```python
from build123d import *

# Parameters (mm, degrees)
F0_W        = 30
F0_H        = 10
F1_DEPTH    = 10
F2_R        = 5
F3_T1_DEPTH = 84.348882825
F4_R        = 10
F5_R        = 50
F6_SIZE     = 2
F8_DEPTH    = 10.001
F9_SIZE     = 2


# Not quite as in the source:
# - a fillet or chamfer that OpenCascade refuses, or shapes differently, is made with other operations: its cross-section is extruded or revolved along the edge and cut away or added


with BuildPart() as f1:
    # F0 (on Top) → F1 (new body)
    with BuildSketch(Plane.XY):
        Polygon((5, 50), (-5, 50), (-15, 65), (-15, 75), (-25, 75), (-25, 61.9722436227), (-5, 31.9722436227), (-5, -50), (5, -50), (5, 31.9722436227), (25, 61.9722436227), (25, 75), (15, 75), (15, 65), align=None)
        with Locations((0, 70)):
            Rectangle(F0_W, F0_H)
    extrude(amount=F1_DEPTH)

    # F2
    f2_edges = [f1.edges().sort_by_distance(p)[0] for p in [
        (15, 65, 5),
        (-15, 65, 5),
        (-5, 50, 5),
        (5, 50, 5),
    ]]
    fillet(f2_edges, radius=F2_R)

    # F3: fillet of radius 15 on 2 edges, made by hand

    # F3_s2 → F3_t1 (cut)
    with BuildSketch(Plane.XY.offset(-37.1744414125)):
        with BuildLine():
            ThreePointArc((-25, 61.9722436227), (-20.0149678844, 71.2823679771), (-10.130223435, 75))
            Line((-10.130223435, 75), (-25, 75))
            Line((-25, 75), (-25, 61.9722436227))
        make_face()
        with BuildLine():
            ThreePointArc((25, 61.9722436227), (20.0149678844, 71.2823679771), (10.130223435, 75))
            Line((10.130223435, 75), (25, 75))
            Line((25, 75), (25, 61.9722436227))
        make_face()
    extrude(amount=F3_T1_DEPTH, mode=Mode.SUBTRACT)

    # F4
    f4_edges = [f1.edges().sort_by_distance(p)[0] for p in [
        (-25, 61.972244, 5),
        (25, 61.972244, 5),
    ]]
    fillet(f4_edges, radius=F4_R)

    # F5
    f5_edges = [f1.edges().sort_by_distance(p)[0] for p in [
        (5, 31.972244, 5),
        (-5, 31.972244, 5),
    ]]
    fillet(f5_edges, radius=F5_R)

    # F6
    f6_edges = [f1.edges().sort_by_distance(p)[0] for p in [
        (0, 65, 10),
        (0, 75, 10),
        (0, 50, 0),
        (0, 75, 0),
    ]]
    chamfer(f6_edges, length=F6_SIZE)

    # F7 (on face) → F8 (cut, through all)
    with BuildSketch(Plane.XY.offset(10)):
        Polygon((0, 37.3431457505), (2.8284271247, 40.1715728753), (0, 43), (-2.8284271247, 40.1715728753), align=None)
    extrude(amount=-F8_DEPTH, mode=Mode.SUBTRACT)

    # F9
    f9_edges = [f1.edges().sort_by_distance(p)[0] for p in [
        (1.414214, 41.585786, 10),
        (-1.414214, 41.585786, 10),
        (1.414214, 38.757359, 10),
        (-1.414214, 38.757359, 10),
        (1.414214, 38.757359, 0),
        (1.414214, 41.585786, 0),
        (-1.414214, 41.585786, 0),
        (-1.414214, 38.757359, 0),
    ]]
    chamfer(f9_edges, length=F9_SIZE)


solid = f1.part
```
Geometry: final body of the model. Coordinates: model frame, mm. A direction names the side the tool comes from. Round coordinates to 2 decimals unless told otherwise and drop trailing zeros. Order: outer loops, then holes, each group sorted by start corner. A loop starts at its lowest first (then second) coordinate and runs counter-clockwise, first axis right, second up. Notation, with made-up numbers: (60, 23.5) -> (80, 23.5) arc R13 ccw to (80, 34.5) -> close; hole circle Ø4 at (-25, 13). An arc over 180 degrees is marked (long way). Use one line per item in the form item = value.
(1) Ray query, probe 1 along X at (y, z) = (-9, 4); probe 2 along Y at (x, z) = (-9, 8.5); probe 3 along X at (y, z) = (57, 4). Return the intervals inside material, ascending. Write a range as [from, to].
Results list:
probe_1 = [-5, 5]
probe_2 = [37.67, 55.1], [64.37, 74.5]
probe_3 = [-21.69, -9.67], [9.67, 21.69]
(2) Section B-B on y = -3.5. Return loops of the section in (x, z).
Results list:
outline = (-5, 2) -> (-3, 0) -> (3, 0) -> (5, 2) -> (5, 8) -> (3, 10) -> (-3, 10) -> (-5, 8) -> close
(3) Draft query along X for faces 1 (the face through (23.845, 64.085, 5.042)), 2 (the face through (-6.69, 31.68, 1.46)), 3 (the face through (2.23, 37.86, 0.79)). Return one class per face: pulls with the +X half, pulls with the -X half, needs draft (parallel to the pull), parting line crosses it, or undercut.
Results list:
face_1 = pulls with the +X half
face_2 = pulls with the -X half
face_3 = undercut
(4) Access query for faces 4 (the face through (1.394, 38.738, 5.042)), 5 (the face through (-2.2, 42.5, 0.8)), 6 (the face through (-2.2, 42.5, 9.2)). Directions: +Z, -Z, +X, -X, +Y, -Y. A direction counts if a zero-diameter tool reaches every point of the face in a straight line with its end or side. Return the directions, or none.
Results list:
face_4 = +Z, -Z
face_5 = -Z
face_6 = +Z
(5) First-contact query: pin 1 Ø5 at (y, z) = (-30, 6) entering from +X; pin 2 Ø6 at (y, z) = (24.5, 8.5) entering from -X; pin 3 Ø5 at (y, z) = (-21, 4.5) entering from -X. Flat tips, straight axial feed; report the tip coordinate or a pass-through.
Results list:
pin_1 = 5
pin_2 = -6.14
pin_3 = -5
(6) Section A-A on z = 4.5. Return loops of the section in (x, y), and give its area (3 significant figures).
Results list:
outline = (-22.2, 57.77) -> (-13.4, 44.57) arc R50 cw to (-5, 16.83) -> (-5, -50) -> (5, -50) -> (5, 16.83) arc R50 cw to (13.4, 44.57) -> (22.2, 57.77) arc R10 ccw to (21.37, 69.94) arc R15 ccw to (10.13, 75) -> (-10.13, 75) arc R15 ccw to (-21.37, 69.94) arc R10 ccw to start; hole (-9.82, 57.23) -> (-6.48, 52.23) arc R5 ccw to (-2.32, 50) -> (2.32, 50) arc R5 ccw to (6.48, 52.23) -> (9.82, 57.23) arc R5 ccw to (5.66, 65) -> (-5.66, 65) arc R5 ccw to start; hole (-2.83, 40.17) -> (0, 37.34) -> (2.83, 40.17) -> (0, 43) -> close
area = 2,040 mm^2
